Source: CAD feature listing. Evaluate the final solid. Frame: model axes, mm. Give positions to 0.01 mm unless a question says otherwise; leave off trailing zeros. Write each loop counter-clockwise with the first axis right and the second up, starting at its lowest first coordinate (ties: lowest second). Pieces come first, ordered by that corner, then holes. Notation, with made-up numbers: (36, -9) -> (60, -9) arc R19 cw to (60, 14) -> close; hole circle Ø5 at (31.5, -9). An arc over 180 degrees is marked (long way). Answer as a JSON object with one key per item and string values. Group by question number.
Item 1: Section query C-C on x = 0. Return the cut outline in (y, z).
Item 2: First-contact query: pin 1 Ø1.6 at (y, z) = (-1.5, 25.5) entering from -X; pin 2 Ø0.8 at (x, z) = (5, 40) entering from +Y; pin 3 Ø6 at (x, z) = (-7.5, 18.5) entering from +Y. Flat tips, straight axial feed; report the tip coordinate or a pass-through.
Item 3: Ray query, probe 1 along X at (y, z) = (1.5, 16); probe 2 along X at (y, z) = (1.25, 58); probe 3 along Y at (x, z) = (-0.75, 21). Return the intervals inside material, ascending. Write a range as from..to.
Item 4: Section query B-B on z = 88.5. Give the number of separate pieces and of enclosed holes in the cut face, plus the area to 3 significant figures.
Item 5: Section query A-A on y = 0. Return the cut outline in (x, z).
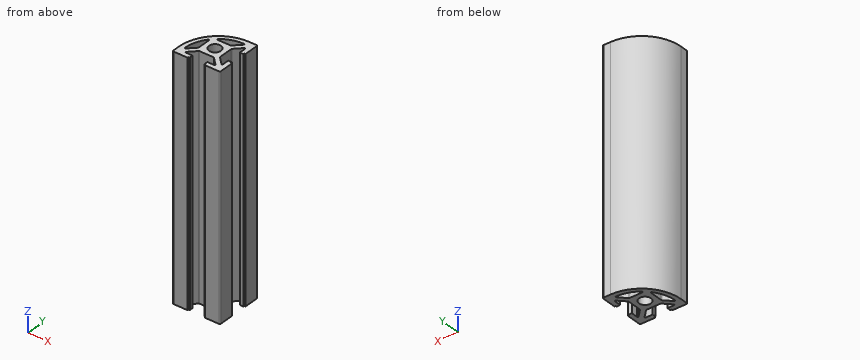
Autodesk Inventor part; units mm, degrees
ref_plane "YZ Plane" through (0, 0, 0) normal (1, 0, 0) x (0, 1, 0)
ref_plane "XZ Plane" through (0, 0, 0) normal (0, 1, 0) x (-1, 0, 0)
ref_plane "XY Plane" through (0, 0, 0) normal (0, 0, 1) x (1, 0, 0)
sketch "Esboço1" plane through (0, 0, 0) normal (0, 0, 1) x (1, 0, 0)
  circle A0 centre (0, 0) radius 2.5
  line L0 (-10, 10) -> (10, 10) construction
  line L1 (10, 10) -> (10, 3.1) construction
  line L2 (8, 3.1) -> (10, 3.1) construction
  line L3 (10, 10) -> (0, 0) construction
  line L4 (-4.5, 4.5) -> (4.5, 4.5) construction
  line L5 (10, -3.1) -> (10, -10) construction
  line L6 (8, -3.1) -> (10, -3.1) construction
  line L7 (4.5, 4.5) -> (4.5, -4.5) construction
  line L8 (-4.5, -4.5) -> (4.5, -4.5) construction
  line L9 (-4.5, 4.5) -> (-4.5, -4.5) construction
  line L10 (8, 6.5858) -> (4.5, 3.0858) construction
  line L11 (8, 6.5858) -> (8, 3.1) construction
  line L12 (0, 0) -> (10, -10) construction
  line L13 (4.5, -3.0858) -> (8, -6.5858) construction
  line L14 (8, -3.1) -> (8, -6.5858) construction
  line L15 (3.0858, -4.5) -> (6.5858, -8) construction
  line L16 (3.1, -10) -> (10, -10) construction
  line L17 (3.1, -8) -> (3.1, -10) construction
  line L18 (3.1, -8) -> (6.5858, -8) construction
  line L19 (0, 0) -> (-10, -10) construction
  line L20 (-10, -10) -> (-3.1, -10) construction
  line L21 (-3.1, -8) -> (-3.1, -10) construction
  line L22 (-3.0858, -4.5) -> (-6.5858, -8) construction
  line L23 (-6.5858, -8) -> (-3.1, -8) construction
  line L24 (-4.5, -3.0858) -> (-8, -6.5858) construction
  arc A1 (-2.8787, -4.5) -> (-3.2322, -4.6464) centre (-2.8787, -5) ccw
  arc A2 (3.2322, -4.6464) -> (2.8787, -4.5) centre (2.8787, -5) ccw
  line L25 (-2.8787, -4.5) -> (2.8787, -4.5)
  line L26 (-3.2322, -4.6464) -> (-6.5858, -8) construction
  arc A3 (4.5, -2.8787) -> (4.6464, -3.2322) centre (5, -2.8787) ccw
  arc A4 (4.6464, 3.2322) -> (4.5, 2.8787) centre (5, 2.8787) ccw
  line L27 (-10, 10) -> (0, 0) construction
  line L28 (4.6464, 3.2322) -> (8, 6.5858) construction
  arc A5 (7.4879, -6.0737) -> (8, -5.8615) centre (7.7, -5.8615) ccw
  line L29 (7.4879, -6.0737) -> (4.6464, -3.2322)
  line L30 (8, -5.8615) -> (8, -3.1)
  arc A6 (5.8615, -8) -> (6.0737, -7.4879) centre (5.8615, -7.7) ccw
  line L31 (5.8615, -8) -> (3.1, -8)
  line L32 (6.0737, -7.4879) -> (3.2322, -4.6464)
  arc A7 (8, 5.8615) -> (7.4879, 6.0737) centre (7.7, 5.8615) ccw
  line L33 (7.4879, 6.0737) -> (4.6464, 3.2322)
  line L34 (8, 5.8615) -> (8, 3.1)
  line L35 (10, 3.1) -> (9.5, 3.1) construction
  line L36 (9.5, 3.1) -> (9.5, 3.6)
  line L37 (9.5, 3.6) -> (10, 3.6)
  line L38 (10, 3.6) -> (10, 3.1) construction
  line L39 (9.5, 3.1) -> (8, 3.1)
  line L40 (10, -3.1) -> (9.5, -3.1) construction
  line L41 (9.5, -3.1) -> (9.5, -3.6)
  line L42 (9.5, -3.6) -> (10, -3.6)
  line L43 (10, -3.6) -> (10, -3.1) construction
  line L44 (9.5, -3.1) -> (8, -3.1)
  line L45 (10, -3.6) -> (10, -10) construction
  line L46 (3.1, -10) -> (3.6, -10) construction
  line L47 (3.6, -10) -> (3.6, -9.5)
  line L48 (3.6, -9.5) -> (3.1, -9.5)
  line L49 (3.1, -9.5) -> (3.1, -10) construction
  line L50 (3.1, -8) -> (3.1, -9.5)
  line L51 (3.6, -10) -> (10, -10) construction
  line L52 (4.5, 2.8787) -> (4.5, -2.8787)
  line L53 (10, 10) -> (10, 3.6) construction
  line L54 (-4.5, 3.086) -> (-4.5, -3.0858) construction
  line L55 (6.5858, 8) -> (3.0858, 4.5) construction
  line L56 (3.0858, 4.5) -> (-3.086, 4.5)
  line L57 (-10, 10) -> (-10, -10) construction
  arc A8 (6.5858, 10) -> (-10, -6.5858) centre (6.5858, -6.5858) ccw
  arc A9 (6.5858, 8) -> (-8, -6.5858) centre (5.9872, -5.9872) ccw construction
  arc A10 (-4.5, 2.4583) -> (-5.0362, 2.6432) centre (-4.8, 2.4583) ccw
  arc A11 (-8.0123, -5.8714) -> (-7.5002, -6.086) centre (-7.7123, -5.8739) ccw
  arc A12 (-5.0362, 2.6432) -> (-8.0123, -5.8714) centre (5.9872, -5.9872) ccw
  arc A13 (-4.6464, -3.2322) -> (-4.5, -2.8787) centre (-5, -2.8787) ccw
  line L58 (-4.5, 2.4583) -> (-4.5, -2.8787)
  line L59 (-7.5002, -6.086) -> (-4.6464, -3.2322)
  line L60 (-10, -6.5858) -> (-10, -10) construction
  line L61 (6.5858, 10) -> (10, 10) construction
  arc A14 (-6.0737, -7.4879) -> (-5.8615, -8) centre (-5.8615, -7.7) ccw
  arc A15 (-2.6432, 5.0362) -> (-2.4583, 4.5) centre (-2.4583, 4.8) ccw
  arc A16 (6.086, 7.5002) -> (5.8714, 8.0123) centre (5.8739, 7.7123) ccw
  arc A17 (2.8787, 4.5) -> (3.2322, 4.6464) centre (2.8787, 5) ccw
  arc A18 (5.8714, 8.0123) -> (-2.6432, 5.0362) centre (5.9872, -5.9872) ccw
  line L62 (3.2322, 4.6464) -> (6.086, 7.5002)
  line L63 (-3.2322, -4.6464) -> (-6.0737, -7.4879)
  line L64 (-5.8615, -8) -> (-3.1, -8)
  line L65 (-3.1, -10) -> (-3.6, -10) construction
  line L66 (-3.6, -10) -> (-3.6, -9.5)
  line L67 (-3.6, -9.5) -> (-3.1, -9.5)
  line L68 (-3.1, -9.5) -> (-3.1, -10) construction
  line L69 (-3.1, -8) -> (-3.1, -9.5)
  line L70 (-10, -10) -> (-3.6, -10) construction
  arc A19 (-10, -9.5) -> (-9.5, -10) centre (-9.5, -9.5) ccw
  line L71 (-10, -6.5858) -> (-10, -9.5)
  line L72 (-9.5, -10) -> (-3.6, -10)
  arc A20 (9.5, -10) -> (10, -9.5) centre (9.5, -9.5) ccw
  line L73 (10, -3.6) -> (10, -9.5)
  line L74 (3.6, -10) -> (9.5, -10)
  arc A21 (10, 9.5) -> (9.5, 10) centre (9.5, 9.5) ccw
  line L75 (10, 9.5) -> (10, 3.6)
  line L76 (6.5858, 10) -> (9.5, 10)
  point P0 (0, 10)
  point P1 (-4.5, 0)
  point P2 (-6.55, -10)
  point P3 (2.8787, 4.5)
  point P4 (-2.4583, 4.5)
  dimension "d0" = 5
  dimension "d1" = 20
  dimension "d2" = 10
  dimension "d4" = 6.9
  dimension "d5" = 2
  dimension "d6" = 2
  dimension "d7" = 6.2
  dimension "d8" = 1
  dimension "d12" = 1
  dimension "d13" = 1
  dimension "d14" = 1
  dimension "d15" = 0.5
  dimension "d16" = 0.5
  dimension "d17" = 0.5
  dimension "d18" = 0.5
  dimension "d19" = 0.3
  dimension "d20" = 0.3
  dimension "d21" = 0.3
  dimension "d22" = 0.5
  dimension "d28" = 1.414
  dimension "d30" = 1
  dimension "d31" = 1.414
  dimension "d34" = 0.3
  dimension "d36" = 0.3
  dimension "d37" = 14
  dimension "d38" = 0.5
  dimension "d39" = 0.3
  dimension "d40" = 0.3
  dimension "d41" = 0.3
  dimension "d42" = 0.5
  dimension "d43" = 0.5
  dimension "d44" = 0.5
  dimension "d45" = 0.5
extrude "Extrusão1" add sketch "Esboço1" along normal blind 100
equation "\"d12\" = d8"
equation "\"d16\" = d15"
equation "\"d17\" = d15"
equation "\"d18\" = d15"
equation "\"d30\" = d8"
equation "\"d31\" = d28"
properties part number "Perfil_20×20_R90_001"
Worked answers:
{
 "1": {"outline": "(-4.5, 0) -> (-2.5, 0) -> (-2.5, 100) -> (-4.5, 100) -> close; (2.5, 0) -> (4.5, 0) -> (4.5, 100) -> (2.5, 100) -> close; (6.67, 0) -> (8.64, 0) -> (8.64, 100) -> (6.67, 100) -> close"},
 "2": {"pin 1": "x = -9.44", "pin 2": "y = 9.96", "pin 3": "y = 5.75"},
 "3": {"probe 1": "-7.9..-5.84, -4.5..-2, 2..4.5", "probe 2": "-8.03..-6, -4.5..-2.17, 2.17..4.5", "probe 3": "-4.5..-2.38, 2.38..4.5, 6.29..8.29"},
 "4": {"separate pieces": "1", "enclosed holes": "3", "area": "192 mm^2"},
 "5": {"outline": "(-8.64, 0) -> (-6.67, 0) -> (-6.67, 100) -> (-8.64, 100) -> close; (-4.5, 0) -> (-2.5, 0) -> (-2.5, 100) -> (-4.5, 100) -> close; (2.5, 0) -> (4.5, 0) -> (4.5, 100) -> (2.5, 100) -> close"}
}
